Work out the finished part from the listing and answer in its coordinate system (mm). A direction names the side the tool comes from. Give positions to 0.01 mm unless a question says otherwise; leave off trailing zeros. Loops run counter-clockwise (first coordinate to the right, second up) from the corner with the lowest first, then second, coordinate; pieces in that order, holes last. Notation, with made-up numbers: M -26,53 L -9,53 A9 ccw -9,63 Z; hole C 74,52 d10. An arc over 180 degrees is marked long. Write item = value, one per line. Start each with the question number.
1. Section A-A on y = -2 is taken. Determine the outline of the cut face in (x, z), plus the area to 3 significant figures.
2. Section D-D on x = 21.5 is taken. Determine the outline of the cut face in (y, z).
3. The mould has two halves that part along Y. Classify faces 3 (the face through (29.544, -11.873, 2.465)), 4 (the face through (6, -8, 5)), 5 (the face through (-13.376, -3.186, 17.325)), 6 (the face through (-14.375, -3.142, 17.325)): released by +Y, released by -Y, zero draft, split by the parting line, or undercut.
4. Section B-B on z = 11 is taken. Determine the outline of the cut face in (x, y), plus the area to 3 significant figures.
5. For faces 1 (the face through (6, 6.623, 2)), 2 (the face through (-9, -3, 5)), determine the directions among +Z, -Z, +X, -X, +Y, -Y from which every point of the face is accessible in a straight line to the end or side of a thin tool.
6. Consider L1, parallel to X at y = -3.25, z = 14; L2, parallel to X at y = -5.75, z = 12.25; L3, parallel to Y at x = 21, z = 14.5. Determine where each line is inside the solid, lowest interval first. Write a range as [from, to].
7. Section C-C on z = 3.5 is taken. Determine the outline of the cut face in (x, y), plus the area to 3 significant figures.
8. Flat-ended cylindrical pins translate along their axes: pin 1 Ø6 at (x, y) = (3, -11) entering from +Z; pin 2 Ø6 at (y, z) = (-2, 26) entering from +X; pin 3 Ø6 at (y, z) = (3, 23) entering from +X. Find the tip coordinate at first contact, or state that the pin passes through.
```python
from build123d import *

# Parameters (mm, degrees)
SKETCH1_R           = 4.85
SKETCH1_R_2         = 3
BOSS_EXTRUDE5_DEPTH = 5
SKETCH1_7_R         = 4.85
BOSS_EXTRUDE6_DEPTH = 5
SKETCH1_8_R         = 5.35
SKETCH1_8_R_2       = 4.35
EXTRUDE_THIN1_DEPTH = 30


with BuildPart() as part:
    # Sketch1 → Boss-Extrude5 (new body)
    with BuildSketch(Plane.XY):
        with BuildLine():
            Line((-14.029850746, 6.623134328), (25.970149254, 6.623134328))
            ThreePointArc((25.970149254, 6.623134328), (29.50568316, 5.158668234), (30.970149254, 1.623134328))
            Line((30.970149254, 1.623134328), (30.970149254, -8.376865672))
            ThreePointArc((30.970149254, -8.376865672), (29.50568316, -11.912399578), (25.970149254, -13.376865672))
            Line((25.970149254, -13.376865672), (-14.029850746, -13.376865672))
            ThreePointArc((-14.029850746, -13.376865672), (-17.565384652, -11.912399578), (-19.029850746, -8.376865672))
            Line((-19.029850746, -8.376865672), (-19.029850746, 1.623134328))
            ThreePointArc((-19.029850746, 1.623134328), (-17.565384652, 5.158668234), (-14.029850746, 6.623134328))
        make_face()
        with Locations((-9.029850746, -3.376865672)):
            Circle(SKETCH1_R, mode=Mode.SUBTRACT)
        with Locations((20.970149254, -3.376865672)):
            Circle(SKETCH1_R, mode=Mode.SUBTRACT)
        with Locations((5.970149254, -3.376865672)):
            Circle(SKETCH1_R_2, mode=Mode.SUBTRACT)
    extrude(amount=BOSS_EXTRUDE5_DEPTH)

    # Sketch1<7> → Boss-Extrude6 (add)
    with BuildSketch(Plane.XY):
        with Locations((-9.029850746, -3.376865672)):
            Circle(SKETCH1_7_R)
        with Locations((20.970149254, -3.376865672)):
            Circle(SKETCH1_7_R)
    extrude(amount=BOSS_EXTRUDE6_DEPTH)

    # Sketch1<8> → Extrude-Thin1 (add)
    with BuildSketch(Plane.XY):
        with Locations((-9.029850746, -3.376865672)):
            Circle(SKETCH1_8_R)
        with Locations((-9.029850746, -3.376865672)):
            Circle(SKETCH1_8_R_2, mode=Mode.SUBTRACT)
        with Locations((20.970149254, -3.376865672)):
            Circle(SKETCH1_8_R)
        with Locations((20.970149254, -3.376865672)):
            Circle(SKETCH1_8_R_2, mode=Mode.SUBTRACT)
    extrude(amount=EXTRUDE_THIN1_DEPTH)


solid = part.part
```
Verdict:
q1.outline = M -19.03,0 L 3.3,0 L 3.3,5 L -3.86,5 L -3.86,30 L -4.9,30 L -4.9,5 L -13.16,5 L -13.16,30 L -14.2,30 L -14.2,5 L -19.03,5 Z; M 8.64,0 L 30.97,0 L 30.97,5 L 26.14,5 L 26.14,30 L 25.1,30 L 25.1,5 L 16.84,5 L 16.84,30 L 15.8,30 L 15.8,5 L 8.64,5 Z
q1.area = 328 mm2
q2.outline = M -13.38,0 L 6.62,0 L 6.62,5 L 1.95,5 L 1.95,30 L 0.94,30 L 0.94,5 L -7.69,5 L -7.69,30 L -8.7,30 L -8.7,5 L -13.38,5 Z
q3.face_3 = released by -Y
q3.face_4 = zero draft
q3.face_5 = undercut
q3.face_6 = split by the parting line
q4.outline = C -9.03,-3.38 d10.7; C 20.97,-3.38 d10.7; hole C -9.03,-3.38 d8.7; hole C 20.97,-3.38 d8.7
q4.area = 60.9 mm2
q5.face_1 = +Z, -Z, +X, -X, +Y
q5.face_2 = +Z
q6.L1 = [-14.38, -13.38], [-4.68, -3.68], [15.62, 16.62], [25.32, 26.32]
q6.L2 = [-13.82, -12.68], [-5.38, -4.23], [16.18, 17.32], [24.62, 25.77]
q6.L3 = [-8.73, -7.73], [0.97, 1.97]
q7.outline = M -19.03,-8.38 A5 ccw -14.03,-13.38 L 25.97,-13.38 A5 ccw 30.97,-8.38 L 30.97,1.62 A5 ccw 25.97,6.62 L -14.03,6.62 A5 ccw -19.03,1.62 Z; hole C 5.97,-3.38 d6
q7.area = 950 mm2
q8.pin_1 = 5
q8.pin_2 = 26.32
q8.pin_3 = 25.12
